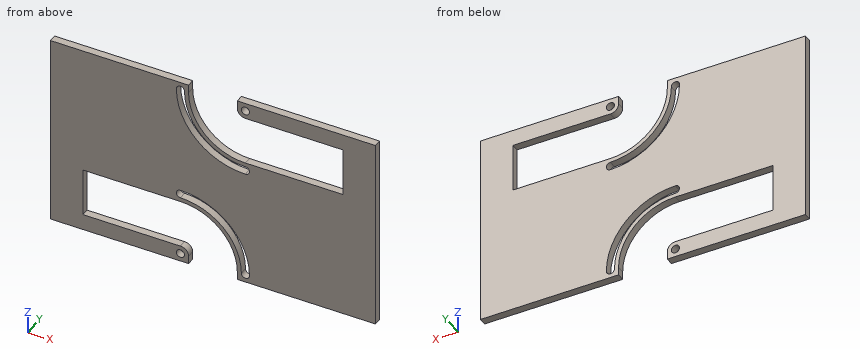
from build123d import *

# Parameters (mm, degrees)
SKETCH2_W           = 127
SKETCH2_H           = 76.2
BOSS_EXTRUDE1_DEPTH = 2.9718
SKETCH3_R           = 1.5875
CUT_EXTRUDE1_DEPTH  = 2.9718
CIRPATTERN1_COUNT   = 2


with BuildPart() as part:
    # Sketch2 → Boss-Extrude1 (new body)
    with BuildSketch(Plane(origin=(0, 0, 0), x_dir=(1, 0, 0), z_dir=(0, 1, 0))):
        Rectangle(SKETCH2_W, SKETCH2_H)
    extrude(amount=BOSS_EXTRUDE1_DEPTH)

    # Sketch3 → Cut-Extrude1 (cut)
    with BuildSketch(Plane(origin=(0, 2.9718, 0), x_dir=(1, 0, 0), z_dir=(0, 1, 0))):
        with BuildLine():
            ThreePointArc((12.7, -12.7), (-3.015448212, -19.209551788), (-9.525, -34.925))
            Line((-9.525, -34.925), (-9.525, -38.1))
            Line((-9.525, -38.1), (9.525, -38.1))
            Line((9.525, -38.1), (9.525, -34.925))
            ThreePointArc((9.525, -34.925), (10.45493597, -32.67993597), (12.7, -31.75))
            Line((12.7, -31.75), (50.8, -31.75))
            Line((50.8, -31.75), (50.8, -12.7))
            Line((50.8, -12.7), (12.7, -12.7))
        make_face()
        with Locations((12.7, -34.925)):
            Circle(SKETCH3_R)
        with BuildLine():
            ThreePointArc((12.7, -7.9375), (-6.383044257, -15.841955743), (-14.2875, -34.925))
            ThreePointArc((-14.2875, -34.925), (-12.7, -36.5125), (-11.1125, -34.925))
            ThreePointArc((-11.1125, -34.925), (-4.137980227, -18.087019773), (12.7, -11.1125))
            ThreePointArc((12.7, -11.1125), (14.2875, -9.525), (12.7, -7.9375))
        make_face()
    cut_extrude1 = extrude(amount=-CUT_EXTRUDE1_DEPTH, mode=Mode.SUBTRACT)

    # CirPattern1: Cut-Extrude1 ×2 about axis
    cirpattern1_axis = Axis((0, 0, 0), (0, 1, 0))
    for i in range(1, CIRPATTERN1_COUNT):
        add(cut_extrude1.rotate(cirpattern1_axis, i * 360 / CIRPATTERN1_COUNT), mode=Mode.SUBTRACT)


solid = part.part
Input: part model. Units: mm. Frame: model coordinates. Give positions to 0.01 mm unless a question says otherwise; leave off trailing zeros. Order: outer loops, then holes, each group sorted by start corner. A loop starts at its lowest first (then second) coordinate and runs counter-clockwise, first axis right, second up. Notation, with made-up numbers: (-32.5, -7) - (-4.5, -7) arc R19 cw to (-4.5, -1) - close; hole circle Ø11 at (18.25, -29.75). An arc over 180 degrees is marked (long way). Answer as a JSON object with one key per item and string values. Group by question number.
Q1. First-contact query: pin 1 Ø1.5 at (x, y) = (9.5, 1.5) entering from -Z. Flat tip, straight axial feed; report the tip coordinate or a pass-through.
Q2. Cut plane A-A, the plane x = 49. Output: boundary loops of the cut face in (y, z), then the cut area to 3 significant figures.
Q3. Cut plane B-B, the plane z = 15.5. Output: boundary loops of the cut face in (x, y).
Q4. Line query: probe 1 along Z at (x, y) = (28, 0.3); probe 2 along X at (y, z) = (0.2, -33.5); probe 3 along X at (y, z) = (1.9, 20). Output: solid intervals per line, ascending.
Q5. Cut plane C-C, the plane y = 0.85. Count the separate pieces of the cut face and the enclosed holes in it, then the cut area to 3 significant figures.
Results:
{
 "1": {"pin 1": "z = -38.1"},
 "2": {"outline": "(0, -38.1) - (2.97, -38.1) - (2.97, 12.7) - (0, 12.7) - close; (0, 31.75) - (2.97, 31.75) - (2.97, 38.1) - (0, 38.1) - close", "area": "170 mm^2"},
 "3": {"outline": "(-63.5, 0) - (-6.03, 0) - (-6.03, 2.97) - (-63.5, 2.97) - close; (-1.07, 0) - (1.9, 0) - (1.9, 2.97) - (-1.07, 2.97) - close; (50.8, 0) - (63.5, 0) - (63.5, 2.97) - (50.8, 2.97) - close"},
 "4": {"probe 1": "-38.1 to 12.7, 31.75 to 38.1", "probe 2": "-63.5 to -13.4, -12 to -9.86, 9.48 to 11.07, 14.25 to 63.5", "probe 3": "-63.5 to -9.78, -5.85 to -3.77, 50.8 to 63.5"},
 "5": {"separate pieces": "1", "enclosed holes": "4", "area": "7,060 mm^2"}
}
